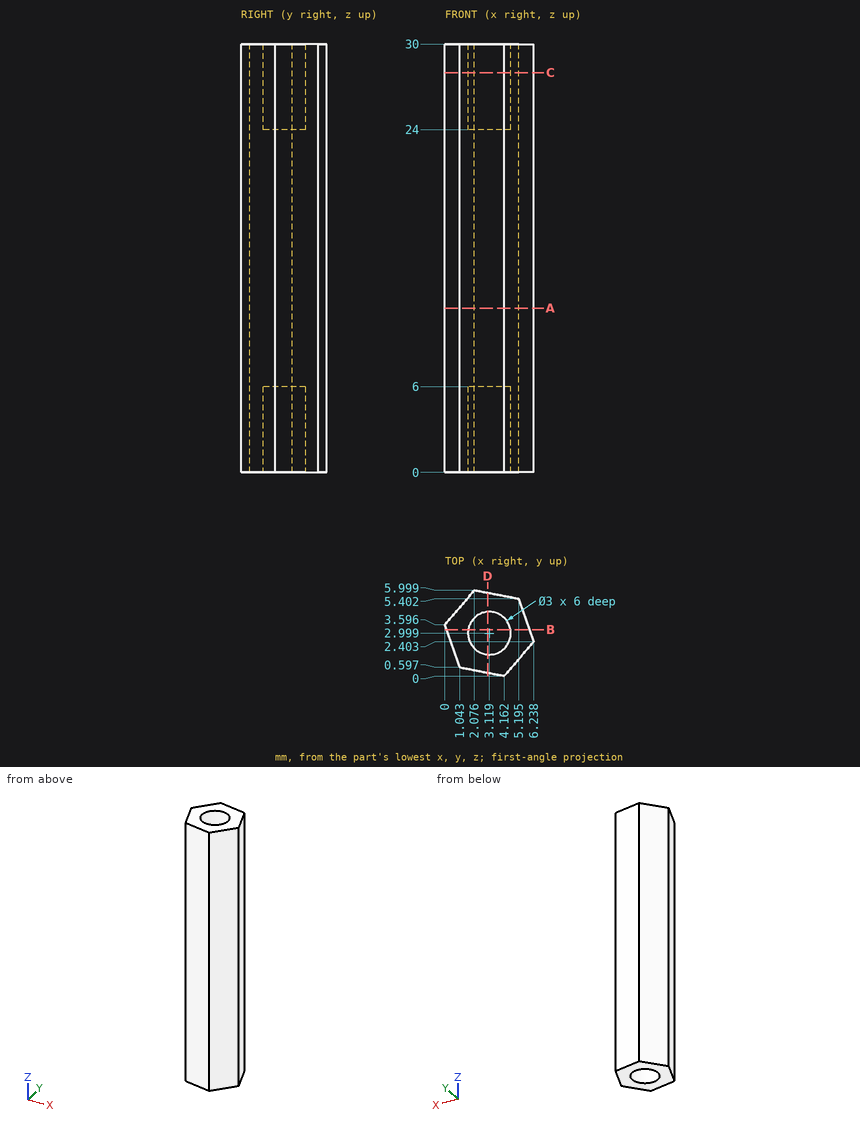
Job drawing, mm, ordinate dimensions from the low corner. One solid piece. Round coordinates to 2 decimals unless told otherwise and drop trailing zeros. Write each loop counter-clockwise with the first axis right and the second up, starting at its lowest first coordinate (ties: lowest second). Pieces come first, ordered by that corner, then holes. Notation, with made-up numbers: (4.5, 7) -> (26.5, 7) arc R23 ccw to (26.5, 21) -> close; hole circle Ø11 at (49.25, 69.5). An arc over 180 degrees is marked (long way). Answer as a JSON object with one key per item and string values.
(1) Probe probe 1 along X at (y, z) = (2.6, 27.5) (1 decimal); probe 2 along X at (y, z) = (5.3, 3.75); probe 3 along Y at (x, z) = (1.75, 22). List the from-to ranges inside material, lowest first. Write a range as [from, to].
Reported:
{"probe 1": "x = [0.3, 1.7], [4.6, 6.2]", "probe 2": "x = [1.47, 5.23]", "probe 3": "y = [0.46, 5.62]"}
(2) Pin check, flat tips, straight feed: P1, Ø1.5, axis at y = 5, z = 18.5, coming from the -X side (1 decimal); P2, Ø1.5, axis at y = 3.5, z = 3.5, coming from the +X side; P3, Ø2.5, axis at x = 3.12, y = 3, coming from the +Z side. Stop position of each tip, or through.
Reported:
{"P1": "stops at x = 0.6", "P2": "stops at x = 6.12", "P3": "stops at z = 24"}
(3) Band-saw the part on B-B, the plane y = 3.25. List the corners of the cut face in (x, z).
Reported:
{"outline": "(0.12, 0) -> (1.64, 0) -> (1.64, 6) -> (4.6, 6) -> (4.6, 0) -> (5.94, 0) -> (5.94, 30) -> (4.6, 30) -> (4.6, 24) -> (1.64, 24) -> (1.64, 30) -> (0.12, 30) -> close"}
(4) Band-saw the part on C-C, the plane z = 28. List the corners of the cut face in (x, y) (1 decimal).
Reported:
{"outline": "(0, 3.6) -> (1, 0.6) -> (4.2, 0) -> (6.2, 2.4) -> (5.2, 5.4) -> (2.1, 6) -> close; hole circle Ø3 at (3.1, 3)"}
(5) Band-saw the part on D-D, the plane x = 3. List the corners of the cut face in (y, z) (1 decimal).
Reported:
{"outline": "(0.2, 0) -> (1.5, 0) -> (1.5, 6) -> (4.5, 6) -> (4.5, 0) -> (5.8, 0) -> (5.8, 30) -> (4.5, 30) -> (4.5, 24) -> (1.5, 24) -> (1.5, 30) -> (0.2, 30) -> close"}
(6) Band-saw the part on A-A, the plane z = 11.5. List the corners of the cut face in (x, y) (1 decimal).
Reported:
{"outline": "(0, 3.6) -> (1, 0.6) -> (4.2, 0) -> (6.2, 2.4) -> (5.2, 5.4) -> (2.1, 6) -> close"}
